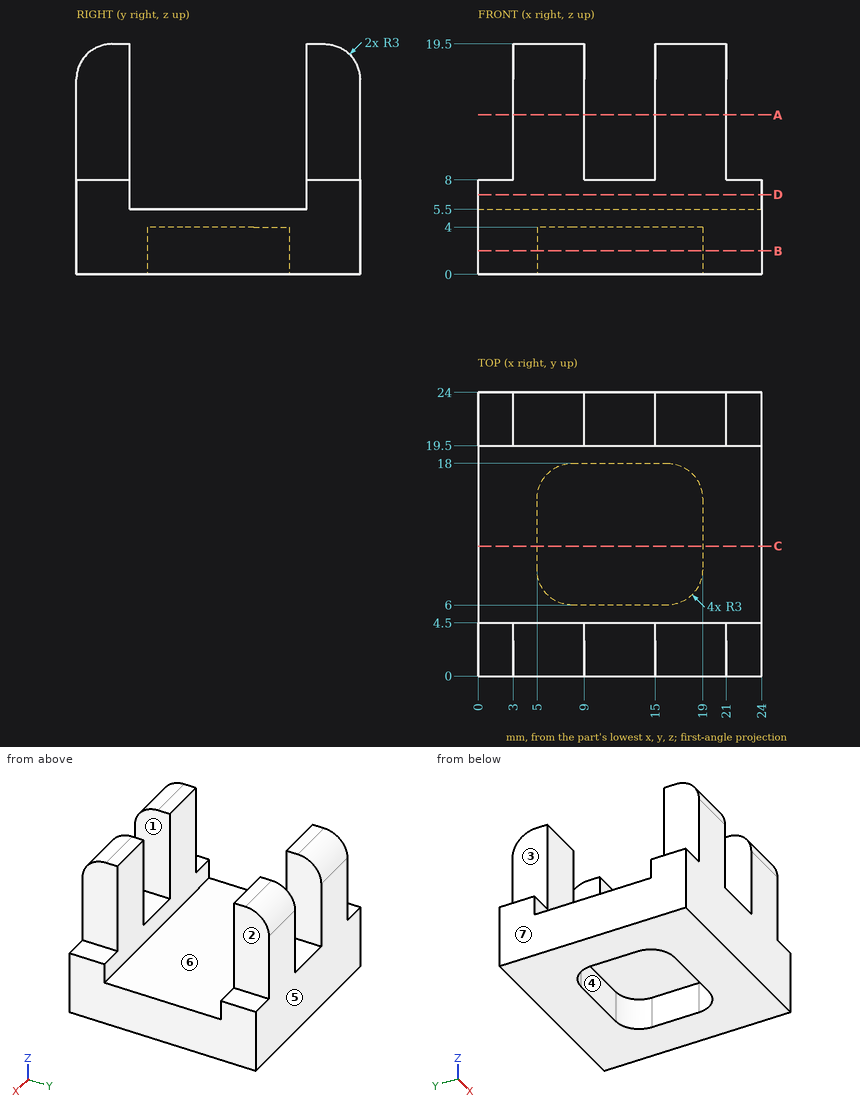
Print and shaded views of the part. All mm, measured from the part's lowest x, y and z. A direction names the side the tool comes from. Round coordinates to 2 decimals unless told otherwise and drop trailing zeros. Order: outer loops, then holes, each group sorted by start corner. A loop starts at its lowest first (then second) coordinate and runs counter-clockwise, first axis right, second up.
Q1. Slice it at C-C (y = 11). Write the cut outline in (x, z).
Q2. Wall check: L1, parallel to X at y = 3.75, z = 14.25; L2, parallel to Y at x = 14.5, z = 7.5; L3, parallel to Z at x = 13.5, y = 13. Give the ranges that are in metal, low to high.
Q3. Slice it at B-B (z = 2). Write the cut outline in (x, y).
Q4. Slice it at D-D (z = 6.75). Write the cut outline in (x, y), and give its area (3 significant figures).
Q5. Two-plate mould, pull along Y, no slides. Class the marked faces 4, 5, 6 and 7: pulls with the +Y half, pulls with the -Y half, needs draft (parallel to the pull), parting line crosses it, or undercut.
Q6. Drop flat-ended pins along their axis: pin 1 (1 mm diameter, centred on y = 13.5, z = 7.5, fed in from +X); pin 2 (1.3 mm diameter, centred on y = 23, z = 12, fed in from +X); pin 3 (3.5 mm diameter, centred on x = 1, y = 1.5, fed in from +Z); pin 4 (4.5 mm diameter, centred on x = 14.5, y = 12.5, fed in from +Z). Give the stop position or say it passes through.
Q7. Which spindle directions (+Z, -Z, +X, -X, +Y, -Y) get a long thin tool onto all of the face, cutting with end or side? Do the marked faces 1, 2 and 3. Say none if no direction does.
Q8. Slice it at A-A (z = 13.5). Write the cut outline in (x, y), and give its area (3 significant figures).
Results below:
1. outline: (0, 0) - (5, 0) - (5, 4) - (19, 4) - (19, 0) - (24, 0) - (24, 5.5) - (0, 5.5) - close
2. L1: x = 3 to 9, 15 to 21
2. L2: y = 0 to 4.5, 19.5 to 24
2. L3: z = 4 to 5.5
3. outline: (0, 0) - (24, 0) - (24, 24) - (0, 24) - close; hole (5, 9) arc R3 ccw to (8, 6) - (16, 6) arc R3 ccw to (19, 9) - (19, 15) arc R3 ccw to (16, 18) - (8, 18) arc R3 ccw to (5, 15) - close
4. outline: (0, 0) - (24, 0) - (24, 4.5) - (0, 4.5) - close; (0, 19.5) - (24, 19.5) - (24, 24) - (0, 24) - close
4. area: 216 mm2
5. face 4: undercut
5. face 5: pulls with the +Y half
5. face 6: undercut
5. face 7: needs draft
6. pin 1: passes through
6. pin 2: stops at x = 21
6. pin 3: stops at z = 8
6. pin 4: stops at z = 5.5
7. face 1: +Z, +Y, -Y
7. face 2: +Z, +X, +Y, -Y
7. face 3: +Z, -X, +Y, -Y
8. outline: (3, 0) - (9, 0) - (9, 4.5) - (3, 4.5) - close; (3, 19.5) - (9, 19.5) - (9, 24) - (3, 24) - close; (15, 0) - (21, 0) - (21, 4.5) - (15, 4.5) - close; (15, 19.5) - (21, 19.5) - (21, 24) - (15, 24) - close
8. area: 108 mm2
